Geometry: final body of the model. Coordinates: model frame, mm. Face numbers are marked on the shaded views. A direction names the side the tool comes from. Round coordinates to 2 decimals unless told otherwise and drop trailing zeros. Loops run counter-clockwise (first coordinate to the right, second up) from the corner with the lowest first, then second, coordinate; pieces in that order, holes last. Notation, with made-up numbers: (-17, 41) - (10, 41) arc R30 cw to (10, 64) - close; hole circle Ø9 at (71, 7). An arc over 180 degrees is marked (long way). Answer as CSV lines item,"result".
from build123d import *

# Parameters (mm, degrees)
BOSS_EXTRUDE1_DEPTH = 6.2
CUT_EXTRUDE1_DEPTH  = 1


with BuildPart() as part:
    # Sketch1 → Boss-Extrude1 (new body)
    with BuildSketch(Plane(origin=(0, 0, 0), x_dir=(-1, 0, 0), z_dir=(0, 0, 1))):
        Polygon((-81.198418694, 94.917906577), (-102.547087364, 86.499465833), (-91.051660388, 81.032468444), (-81.198418694, 84.917906577), (-74.998418694, 84.917906577), (-74.998418694, 94.917906577), align=None)
    extrude(amount=BOSS_EXTRUDE1_DEPTH)

    # Sketch2 → Cut-Extrude1 (cut)
    with BuildSketch(Plane.XY.offset(6.2)):
        with BuildLine():
            Line((83.169030289, -88.057134239), (83.169030289, -88.382775265))
            Line((83.169030289, -88.382775265), (82.089072356, -88.382775265))
            Line((82.089072356, -88.382775265), (81.917983614, -89.217866411))
            add(Edge.make_bspline(
                [(81.917983614, -89.217866411), (81.951598586, -89.208586093), (82.016722277, -89.190606945), (82.112843008, -89.170644567), (82.204094507, -89.158610914), (82.263308593, -89.156967797), (82.291961979, -89.156172701)],
                knots=[0, 0, 0, 0, 0.000104595, 0.000202637, 0.000294305, 0.000380252, 0.000380252, 0.000380252, 0.000380252], degree=3))
            add(Edge.make_bspline(
                [(82.291961979, -89.156172701), (82.327416515, -89.156940085), (82.397128989, -89.158448955), (82.499127177, -89.172937704), (82.596493445, -89.195743198), (82.689024166, -89.227602529), (82.776890523, -89.268342072), (82.859284096, -89.319232733), (82.937441632, -89.378680826), (83.009960985, -89.447029515), (83.075750893, -89.522251268), (83.133595755, -89.603130193), (83.182728962, -89.688880287), (83.222244789, -89.780320839), (83.25379915, -89.876440928), (83.274801317, -89.978251914), (83.288786474, -90.084794137), (83.290348924, -90.157641854), (83.291145673, -90.194789488)],
                knots=[0, 0, 0, 0, 0.000106308, 0.000209029, 0.000308378, 0.000405929, 0.000502102, 0.000598312, 0.00069588, 0.000796219, 0.000896736, 0.000995218, 0.001094066, 0.001192613, 0.001293582, 0.001396995, 0.001504047, 0.001615439, 0.001615439, 0.001615439, 0.001615439], degree=3))
            add(Edge.make_bspline(
                [(83.291145673, -90.194789488), (83.290542355, -90.220663216), (83.289343872, -90.272061012), (83.283249153, -90.348391823), (83.271514611, -90.423106678), (83.255759604, -90.496215491), (83.23531041, -90.56757985), (83.21055534, -90.637404022), (83.180260372, -90.705253415), (83.147030482, -90.771770023), (83.109614034, -90.835450098), (83.068086388, -90.895003107), (83.024211978, -90.95132242), (82.977003007, -91.00380402), (82.926020676, -91.052103044), (82.87188242, -91.096506128), (82.815020239, -91.137764191), (82.754554412, -91.174202483), (82.691832303, -91.207733164), (82.625948134, -91.235240945), (82.558401642, -91.259834067), (82.488220647, -91.279436995), (82.415564117, -91.294797241), (82.340312285, -91.305229929), (82.26285982, -91.312828554), (82.210358916, -91.313304221), (82.183838983, -91.313544496)],
                knots=[0, 0, 0, 0, 7.7636e-05, 0.000154223, 0.000229512, 0.000304362, 0.000378447, 0.000452077, 0.000526407, 0.000601214, 0.00067506, 0.000747747, 0.00081887, 0.000889121, 0.000959302, 0.001029336, 0.001099058, 0.00116985, 0.001240974, 0.00131221, 0.00138383, 0.001456517, 0.001530612, 0.001606437, 0.001684346, 0.001763871, 0.001763871, 0.001763871, 0.001763871], degree=3))
            add(Edge.make_bspline(
                [(82.183838983, -91.313544496), (82.152203119, -91.312917807), (82.089963294, -91.311684871), (81.998776779, -91.298786674), (81.911042816, -91.280313692), (81.827467652, -91.252522219), (81.747302292, -91.217699459), (81.671625969, -91.17368836), (81.598505015, -91.123814459), (81.530911953, -91.06495871), (81.468177479, -91.000628056), (81.412019432, -90.930816481), (81.362005401, -90.856676202), (81.318936302, -90.777847162), (81.282198811, -90.694536495), (81.253338072, -90.606432058), (81.230044136, -90.513994197), (81.220189462, -90.450354942), (81.215184135, -90.418031675)],
                knots=[0, 0, 0, 0, 9.4843e-05, 0.000186593, 0.000275792, 0.000363484, 0.000450342, 0.000537514, 0.000625728, 0.000715478, 0.000805885, 0.000894984, 0.00098389, 0.001073836, 0.001164117, 0.001256635, 0.001351658, 0.001449737, 0.001449737, 0.001449737, 0.001449737], degree=3))
            Line((81.215184135, -90.418031675), (81.500120032, -90.418031675))
            add(Edge.make_bspline(
                [(81.500120032, -90.418031675), (81.507130938, -90.448308886), (81.520606288, -90.506503365), (81.55018436, -90.588265368), (81.586348404, -90.661126378), (81.62935092, -90.726050214), (81.680649876, -90.78266409), (81.739187287, -90.833116711), (81.804817007, -90.878632721), (81.877745151, -90.916571945), (81.95468273, -90.9489286), (82.035207271, -90.970474781), (82.117126214, -90.985624876), (82.172533021, -90.987141402), (82.200375441, -90.98790347)],
                knots=[0, 0, 0, 0, 9.3172e-05, 0.000179081, 0.000260145, 0.000336703, 0.000411917, 0.000488562, 0.000568128, 0.000650923, 0.00073478, 0.000817953, 0.000900557, 0.000983994, 0.000983994, 0.000983994, 0.000983994], degree=3))
            add(Edge.make_bspline(
                [(82.200375441, -90.98790347), (82.22755203, -90.987158907), (82.281062956, -90.985692857), (82.359813285, -90.974408896), (82.435843535, -90.957030242), (82.508403495, -90.931022588), (82.578762891, -90.899413451), (82.645141954, -90.858850489), (82.709460993, -90.812168901), (82.7697208, -90.758686815), (82.824910872, -90.699750021), (82.873675353, -90.636724099), (82.91429441, -90.569489531), (82.948524637, -90.499210314), (82.974517273, -90.425116194), (82.993060163, -90.347554414), (83.003948652, -90.266333396), (83.005446508, -90.210934808), (83.006209776, -90.182705153)],
                knots=[0, 0, 0, 0, 8.15e-05, 0.000160473, 0.000238226, 0.000315066, 0.000391338, 0.000469218, 0.000547964, 0.000629516, 0.000710512, 0.000789892, 0.000868102, 0.000945761, 0.001024012, 0.00110315, 0.001184644, 0.001269321, 0.001269321, 0.001269321, 0.001269321], degree=3))
            add(Edge.make_bspline(
                [(83.006209776, -90.182705153), (83.005612441, -90.157236435), (83.004443243, -90.107385045), (82.994890511, -90.034451479), (82.978274401, -89.965442362), (82.955211309, -89.900024449), (82.925929185, -89.838136041), (82.890145744, -89.779713265), (82.847189447, -89.725526145), (82.798120377, -89.675549328), (82.744364868, -89.629425763), (82.684998045, -89.590106485), (82.621262254, -89.557028502), (82.553925403, -89.528482533), (82.481385817, -89.507980428), (82.405080014, -89.492588132), (82.324184001, -89.483684196), (82.268874876, -89.482448768), (82.240444552, -89.481813727)],
                knots=[0, 0, 0, 0, 7.6388e-05, 0.000149519, 0.000220172, 0.000288967, 0.000357247, 0.000425206, 0.000494043, 0.000564207, 0.000635056, 0.000706145, 0.000777268, 0.000850264, 0.000925136, 0.001002969, 0.001083601, 0.001168886, 0.001168886, 0.001168886, 0.001168886], degree=3))
            add(Edge.make_bspline(
                [(82.240444552, -89.481813727), (82.215834738, -89.482340406), (82.165021715, -89.483427864), (82.087077437, -89.491434758), (82.005169945, -89.504351832), (81.919613224, -89.522119357), (81.830150335, -89.545370405), (81.736970071, -89.573232845), (81.639876515, -89.606544944), (81.574455436, -89.631702023), (81.540825161, -89.644634239)],
                knots=[0, 0, 0, 0, 7.3822e-05, 0.000152423, 0.000234822, 0.000322511, 0.00041445, 0.000512043, 0.000614219, 0.000722306, 0.000722306, 0.000722306, 0.000722306], degree=3))
            Line((81.540825161, -89.644634239), (81.866466186, -88.057134239))
            Line((81.866466186, -88.057134239), (83.169030289, -88.057134239))
        make_face()
        Polygon((85.349934736, -87.975723983), (85.40781234, -87.975723983), (85.40781234, -90.173800906), (85.774158494, -90.173800906), (85.774158494, -90.499441932), (85.40781234, -90.499441932), (85.40781234, -91.232134239), (85.122876443, -91.232134239), (85.122876443, -90.499441932), (83.616786699, -90.499441932), align=None)
        Polygon((85.122876443, -90.173800906), (85.122876443, -88.794914688), (84.176482212, -90.173800906), align=None, mode=Mode.SUBTRACT)
    extrude(amount=-CUT_EXTRUDE1_DEPTH, mode=Mode.SUBTRACT)


solid = part.part
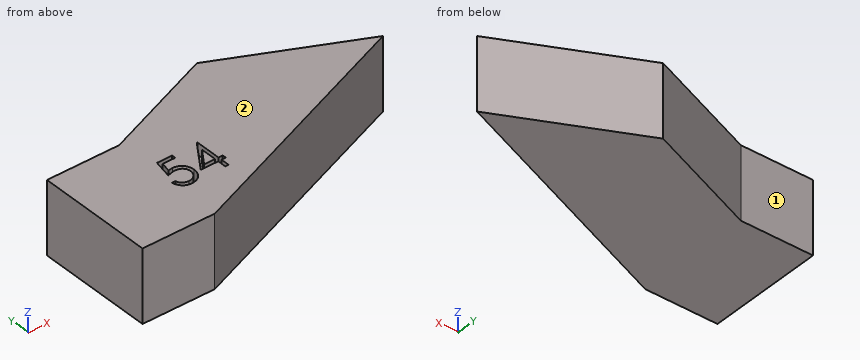
(1) Section D-D (y = -84.25). Output: boundary loops of the cut face in (x, z).
Findings below:
outline,"(82.89, 0) - (97.82, 0) - (97.82, 6.2) - (82.89, 6.2) - close"
(2) Material intervals for line 1 along Y through (x, z) = (78.75, 2.5); line 2 along Y through (x, z) = (97, 2.5), sorted ascending.
Findings below:
line 1,"-94.92 to -84.92"
line 2,"-88.69 to -83.86"
(3) Pin query (flat end, axial travel): P1, Ø0.8, axis at x = 84.5, z = 5.5, coming from the -Y side; P2, Ø0.8, axis at x = 84.5, z = 5.5, coming from the +Y side; P3, Ø1.1, axis at x = 82.5, z = 5.5, coming from the -Y side. Return the tip coordinate at first contact, or that it passes through.
Findings below:
P1,"y = -93.77"
P2,"y = -83.46"
P3,"y = -94.62"
(4) Access query for the marked faces 1 and 2. Directions: +Z, -Z, +X, -X, +Y, -Y. A direction counts if a zero-diameter tool reaches every point of the face in a straight line with its end or side. Return the directions, or none.
Findings below:
face 1,"+Z, -Z, -X, +Y"
face 2,"+Z, +X, -X, +Y, -Y"
(5) Section C-C (x = 84.75). Output: boundary loops of the cut face in (y, z), and give its area (3 significant figures).
Findings below:
outline,"(-93.52, 0) - (-83.52, 0) - (-83.52, 6.2) - (-88.85, 6.2) - (-88.85, 5.2) - (-89.34, 5.2) - (-89.34, 6.2) - (-90.17, 6.2) - (-90.17, 5.2) - (-90.5, 5.2) - (-90.5, 6.2) - (-93.52, 6.2) - close"
area,"61.2 mm2"
(6) Section B-B (z = 4.5). Output: boundary loops of the cut face in (x, y).
Findings below:
outline,"(75, -94.92) - (81.2, -94.92) - (102.55, -86.5) - (91.05, -81.03) - (81.2, -84.92) - (75, -84.92) - close"
(7) Section A-A (z = 5.75). Give the number of separate pieces and of enclosed holes in the cut face, and give its area (3 significant figures).
Findings below:
separate pieces,"2"
enclosed holes,"2"
area,"214 mm2"
